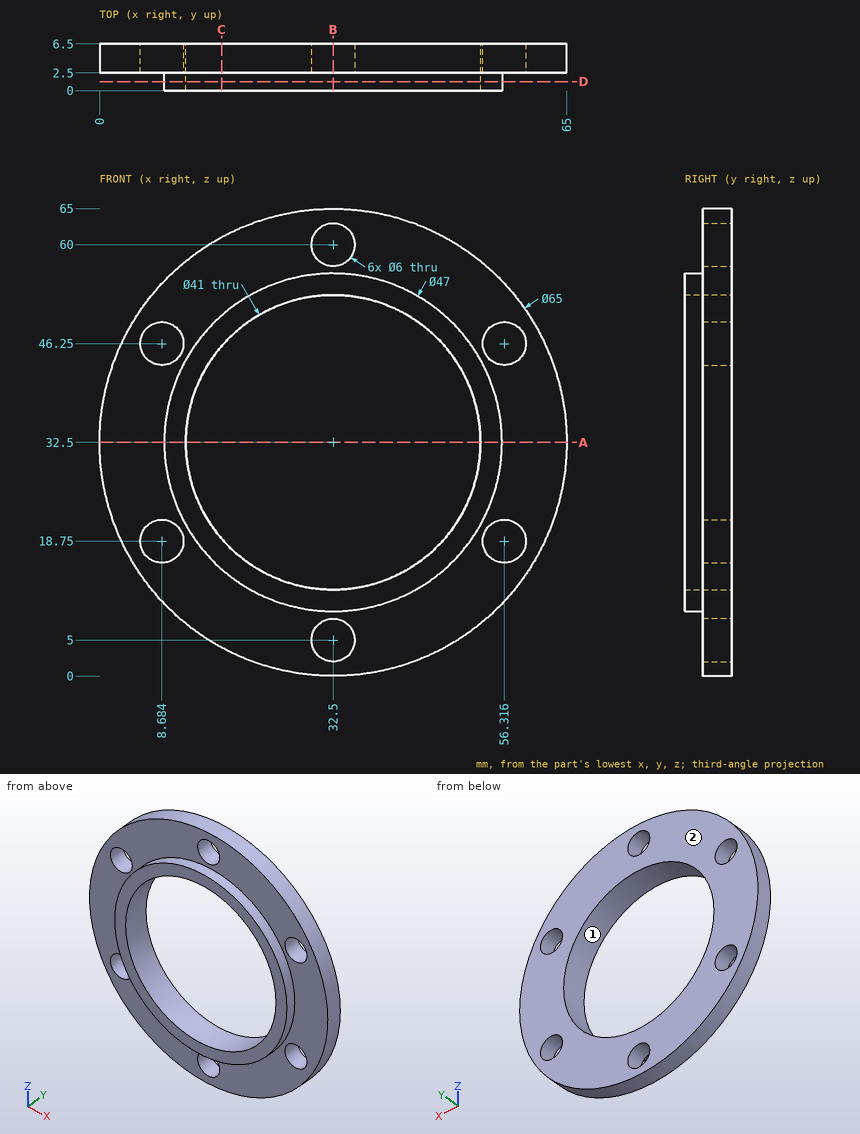
Study the drawing (mm; zero at the part's minimum x, y, z) and answer. Give positions to 0.01 mm unless a question says otherwise; leave off trailing zeros. Write each loop counter-clockwise with the first axis right and the second up, starting at its lowest first coordinate (ties: lowest second). Pieces come first, ordered by that corner, then holes. Notation, with made-up numbers: (71, 31) - (79, 31) arc R17 cw to (79, 42) - close; hole circle Ø3 at (86, 83). An arc over 180 degrees is marked (long way). Use CSV: the item, a comma, the result in double quotes. Start each with the question number.
(1) Given P1, Ø1.5, axis at y = 5.5, z = 9, coming from the +X side; P2, Ø1.5, axis at y = 4, z = 53, coming from the +X side; P3, Ø1, axis at y = 4.5, z = 56, coming from the +X side, each flat-ended and moving along its own axis, determine where each tip first touches the part or whether it passes through.
(2) Find section C-C (x = 17). Give the vertices of the cut face in (y, z).
(3) Determine the mould class of the marked faces 1 and 2 for opening direction Z: +Z half, -Z half, draft (parallel to the pull), parting line (faces both ways), or undercut.
(4) Find section B-B (x = 32.5). Give the vertices of the cut face in (y, z).
(5) Consider line 1 along Z through (x, y) = (32.5, 3.55); line 2 along X through (y, z) = (2.75, 32.5); line 3 along Z through (x, y) = (6, 4) (1 decimal). Determine where each line is inside the solid, lowest interval first.
(6) Find section D-D (y = 1.25). Give the vertices of the cut face in (x, z).
(7) Find section A-A (z = 32.5). Give the vertices of the cut face in (x, y), plus the area to 3 significant figures.
Findings below:
1,P1,"x = 55.71"
1,P2,"x = 58.31"
1,P3,"x = 55.46"
2,outline,"(0, 14.84) - (2.5, 14.84) - (2.5, 3.93) - (6.5, 3.93) - (6.5, 19.08) - (0, 19.08) - close; (0, 45.92) - (6.5, 45.92) - (6.5, 61.07) - (2.5, 61.07) - (2.5, 50.16) - (0, 50.16) - close"
3,face 1,"undercut"
3,face 2,"draft"
4,outline,"(0, 9) - (2.5, 9) - (2.5, 8) - (6.5, 8) - (6.5, 12) - (0, 12) - close; (0, 53) - (6.5, 53) - (6.5, 57) - (2.5, 57) - (2.5, 56) - (0, 56) - close; (2.5, 0) - (6.5, 0) - (6.5, 2) - (2.5, 2) - close; (2.5, 63) - (6.5, 63) - (6.5, 65) - (2.5, 65) - close"
5,line 1,"0 to 2, 8 to 12, 53 to 57, 63 to 65"
5,line 2,"0 to 12, 53 to 65"
5,line 3,"13.7 to 17.4, 20.1 to 44.9, 47.6 to 51.3"
6,outline,"circle Ø47 at (32.5, 32.5); hole circle Ø41 at (32.5, 32.5)"
7,outline,"(0, 2.5) - (9, 2.5) - (9, 0) - (12, 0) - (12, 6.5) - (0, 6.5) - close; (53, 0) - (56, 0) - (56, 2.5) - (65, 2.5) - (65, 6.5) - (53, 6.5) - close"
7,area,"111 mm2"
